from build123d import *
from build123d.topology import SkipClean

# Parameters (mm, degrees)
SKETCH1_R               = 38.1
BOSS_EXTRUDE1_DEPTH     = 76.2
SHELL2_T                = 3.175
BOSS_EXTRUDE2_DEPTH     = 7
CUT_EXTRUDE1_DEPTH      = 99.527366122
CUT_EXTRUDE1_DEPTH_BACK = 99.527366122
SKETCH3_R               = 61.906276858
SKETCH3_R_2             = 41.275
SKETCH4_R               = 20.64
CUT_EXTRUDE2_DEPTH      = 7
SCALE1_SCALE            = 0.615384615


# Read off the part's stored shape, not the designer's step: Boss-Extrude2
with BuildPart() as part:
    # Sketch1 → Boss-Extrude1 (new body)
    with BuildSketch(Plane(origin=(0, 0, 0), x_dir=(1, 0, 0), z_dir=(0, 1, 0))):
        with Locations(Location((0, 0, 0), (0, 0, 90))):
            Circle(SKETCH1_R)
    extrude(amount=BOSS_EXTRUDE1_DEPTH)

    # Shell2
    shell2_openings = [part.faces().sort_by_distance(p)[0] for p in [
        (0, 76.2, 0),
    ]]
    offset(amount=SHELL2_T, openings=shell2_openings, kind=Kind.INTERSECTION)

    # Boss-Extrude2 outline → Boss-Extrude2 (add)
    with BuildSketch(Plane(origin=(0, -3.175, 0), x_dir=(-1, 0, 0), z_dir=(0, -1, 0))):
        Polygon((1.5, 14.271546681), (1.5, 41.275), (-1.5, 41.275), (-1.5, 14.271546681), (-7.114333637, 40.684909757), (-10.04877644, 40.061174684), (-4.434442802, 13.647811609), (-15.417736756, 38.316693729), (-18.158373129, 37.0964838), (-7.175079175, 12.42760168), (-23.047310797, 34.273854321), (-25.47436178, 32.510498564), (-9.602130158, 10.664245923), (-29.669606762, 28.733083016), (-31.676998581, 26.503648539), (-11.609521977, 8.434811446), (-34.995198541, 21.936538106), (-36.495198541, 19.338461894), (-13.109521977, 5.836735235), (-38.791332219, 14.181261217), (-39.718383202, 11.328091668), (-14.03657296, 2.983565686), (-40.892098536, 5.806195164), (-41.205683926, 2.822629478), (-14.35015835, 0), (-41.205683926, -2.822629478), (-40.892098536, -5.806195164), (-14.03657296, -2.983565686), (-39.718383202, -11.328091668), (-38.791332219, -14.181261217), (-13.109521977, -5.836735235), (-36.495198541, -19.338461894), (-34.995198541, -21.936538106), (-11.609521977, -8.434811446), (-31.676998581, -26.503648539), (-29.669606762, -28.733083016), (-9.602130158, -10.664245923), (-25.47436178, -32.510498564), (-23.047310797, -34.273854321), (-7.175079175, -12.42760168), (-18.158373129, -37.0964838), (-15.417736756, -38.316693729), (-4.434442802, -13.647811609), (-10.04877644, -40.061174684), (-7.114333637, -40.684909757), (-1.5, -14.271546681), (-1.5, -41.275), (1.5, -41.275), (1.5, -14.271546681), (7.114333637, -40.684909757), (10.04877644, -40.061174684), (4.434442802, -13.647811609), (15.417736756, -38.316693729), (18.158373129, -37.0964838), (7.175079175, -12.42760168), (23.047310797, -34.273854321), (25.47436178, -32.510498564), (9.602130158, -10.664245923), (29.669606762, -28.733083016), (31.676998581, -26.503648539), (11.609521977, -8.434811446), (34.995198541, -21.936538106), (36.495198541, -19.338461894), (13.109521977, -5.836735235), (38.791332219, -14.181261217), (39.718383202, -11.328091668), (14.03657296, -2.983565686), (40.892098536, -5.806195164), (41.205683926, -2.822629478), (14.35015835, 0), (41.205683926, 2.822629478), (40.892098536, 5.806195164), (14.03657296, 2.983565686), (39.718383202, 11.328091668), (38.791332219, 14.181261217), (13.109521977, 5.836735235), (36.495198541, 19.338461894), (34.995198541, 21.936538106), (11.609521977, 8.434811446), (31.676998581, 26.503648539), (29.669606762, 28.733083016), (9.602130158, 10.664245923), (25.47436178, 32.510498564), (23.047310797, 34.273854321), (7.175079175, 12.42760168), (18.158373129, 37.0964838), (15.417736756, 38.316693729), (4.434442802, 13.647811609), (10.04877644, 40.061174684), (7.114333637, 40.684909757), align=None)
    extrude(amount=BOSS_EXTRUDE2_DEPTH)

    # Sketch3 → Cut-Extrude1 (cut, two sides: drawn at the far end of the back side and taken through both)
    with SkipClean():  # the faces are left unmerged after this step: merging them gives an invalid solid
        with BuildSketch(Plane.XZ.offset(3.175).offset(-CUT_EXTRUDE1_DEPTH_BACK)):
            Circle(SKETCH3_R)
            with Locations(Location((0, 0, 0), (0, 0, 272.082679548))):
                Circle(SKETCH3_R_2, mode=Mode.SUBTRACT)
        extrude(amount=CUT_EXTRUDE1_DEPTH + CUT_EXTRUDE1_DEPTH_BACK, mode=Mode.SUBTRACT)

    # Sketch4 → Cut-Extrude2 (cut)
    with SkipClean():  # the faces are left unmerged after this step: merging them gives an invalid solid
        with BuildSketch(Plane.XZ.offset(10.175)):
            Circle(SKETCH4_R)
        extrude(amount=-CUT_EXTRUDE2_DEPTH, mode=Mode.SUBTRACT)


with BuildPart() as part_1:
    # Scale1: scaled about (0, 24.187012891, 0)
    add(part.part.scale(SCALE1_SCALE).moved(Location((0, 9.302697266, 0))))


solid = part_1.part
For this review, take the finished solid that the model builds, in its own axes (mm). A direction names the side the tool comes from. Coordinates: 2 decimals unless noted, no trailing zeros. Loops run counter-clockwise (first coordinate to the right, second up) from the corner with the lowest first, then second, coordinate; pieces in that order, holes last. Notation, with made-up numbers: (9.25, 86) - (48.25, 86) arc R19 ccw to (48.25, 117) - close; hole circle Ø5 at (56.5, 85.5). An arc over 180 degrees is marked (long way). Return JSON: item names as keys, results as strings.
Item 1: For faces 1 (the cylindrical face through (-12.633, 5.165, -1.315)), 2 (the flat face through (0, 9.303, 0)), 3 (the flat face through (-18, 3.041, -6)), 4 (the flat face through (18.93, 5.23, 1.06)), list the 3-axis set-ups (+Z, -Z, +X, -X, +Y, -Y) from which the entire face can be reached by the end or side of a thin tool; tool diameter is ignored.
Determined:
{"face 1": "-Y", "face 2": "+Y", "face 3": "+Z, -Z, +X, -X, -Y", "face 4": "+X, -Y"}
Item 2: For line 1 (X direction, y = 6.5, z = 23); line 2 (X direction, y = 15, z = 0.5); line 3 (X direction, y = 18, z = -13), list the stretches that pass through material, from the lowest coordinate up.
Determined:
{"line 1": "x = -10.78 to -9.23, -5.83 to -3.95, -0.92 to 0.92, 3.95 to 5.83, 9.23 to 10.78", "line 2": "x = -25.4 to -23.44, 23.44 to 25.4", "line 3": "x = -21.82 to -19.51, 19.51 to 21.82"}
Item 3: Take a section at A-A (y = 36). Give the boundary of the cut face in (x, z).
Determined:
{"outline": "circle Ø50.8 at (0, 0); hole circle Ø46.89 at (0, 0)"}
Item 4: Mouldability with a two-part tool opening along Z and no side actions: class faces 5 (the cylindrical face through (-9.43, 5.16, 8.51)), 6 (the flat face through (14, 3.041, -13)) as pulls with the +Z half, pulls with the -Z half, needs draft (parallel to the pull), parting line crosses it, or undercut.
Determined:
{"face 5": "undercut", "face 6": "needs draft"}
Item 5: Insertion check: pin 1 (1.3 mm diameter, centred on y = 5, z = 16.5, fed in from -X); pin 2 (2 mm diameter, centred on x = -14.5, z = 0.5, fed in from +Y); pin 3 (5 mm diameter, centred on y = 41, z = 20, fed in from -X). Each pin has a flat end and moves straight along its axis. Give the tip position at first contact, or say it passes through.
Determined:
{"pin 1": "stops at x = -19.48", "pin 2": "stops at y = 9.3", "pin 3": "stops at x = -18.41"}
